from build123d import *

# Parameters (mm, degrees)
SKETCH1_W           = 225.40000005
SKETCH1_H           = 111.10000005
SKETCH1_R           = 2.499999953
BOSS_EXTRUDE1_DEPTH = 19.38655
CUT_EXTRUDE1_DEPTH  = 2.54


with BuildPart() as part:
    # Sketch1 → Boss-Extrude1 (new, symmetric)
    with BuildSketch(Plane(origin=(0, 0, 0), x_dir=(1, 0, 0), z_dir=(0, 1, 0))):
        with Locations((112.700000025, 55.550000025)):
            Rectangle(SKETCH1_W, SKETCH1_H)
        with Locations(Location((4.800000052, 4.800000052, 0), (0, 0, 270))):
            Circle(SKETCH1_R, mode=Mode.SUBTRACT)
        with Locations(Location((4.800000052, 106.400000052, 0), (0, 0, 270))):
            Circle(SKETCH1_R, mode=Mode.SUBTRACT)
        with Locations(Location((220.700000052, 106.400000052, 0), (0, 0, 270))):
            Circle(SKETCH1_R, mode=Mode.SUBTRACT)
        with Locations(Location((220.700000052, 4.800000052, 0), (0, 0, 270))):
            Circle(SKETCH1_R, mode=Mode.SUBTRACT)
    extrude(amount=BOSS_EXTRUDE1_DEPTH, both=True)

    # Sketch2 → Cut-Extrude1 (cut)
    # profile 1 of 3: a face of its own
    with BuildSketch(Plane(origin=(0, 19.38655, 0), x_dir=(1, 0, 0), z_dir=(0, 1, 0))):
        with BuildLine():
            add(Edge.make_bspline(
                [(93.6654446, 62.638119725), (93.65621175, 62.255926888), (93.637663033, 61.488104777), (93.466421809, 60.341834085), (93.201255703, 59.201705874), (92.836997723, 58.075217304), (92.359286935, 56.979010165), (91.762331794, 55.932624231), (91.032595392, 54.955716054), (90.207106522, 54.027487516), (89.252652089, 53.179116743), (88.173798237, 52.414727304), (86.973600637, 51.734204765), (85.655660468, 51.128628725), (84.202701193, 50.653409294), (82.618753702, 50.300761726), (80.898189452, 50.099121533), (79.705954978, 50.07473573), (79.09029785, 50.062143162)],
                knots=[0, 0, 0, 0, 0.84837333, 1.704374698, 2.568122001, 3.446177459, 4.329841521, 5.219461111, 6.115085959, 7.03322926, 7.973947317, 8.94447037, 9.964314875, 11.034235969, 12.160282575, 13.352588404, 14.632904974, 16, 16, 16, 16], degree=3))
            Line((79.09029785, 50.062143162), (74.528088962, 50.062143162))
            Line((74.528088962, 50.062143162), (74.528088962, 36.39260342))
            Line((74.528088962, 36.39260342), (69.060273065, 36.39260342))
            Line((69.060273065, 36.39260342), (69.060273065, 74.120533108))
            Line((69.060273065, 74.120533108), (79.611449053, 74.120533108))
            add(Edge.make_bspline(
                [(79.611449053, 74.120533108), (80.070260309, 74.115673927), (80.980958213, 74.106028903), (82.329353652, 73.976911734), (83.651671763, 73.795021467), (84.937147693, 73.523102459), (86.171480276, 73.166358976), (87.344146306, 72.730911072), (88.422755699, 72.162952721), (89.43560104, 71.526521333), (90.368402205, 70.791840353), (91.189022047, 69.939252772), (91.912770344, 68.989458848), (92.539599198, 67.944691466), (93.055694596, 66.787250357), (93.402550005, 65.504823346), (93.635402669, 64.110350409), (93.655195832, 63.140369447), (93.6654446, 62.638119725)],
                knots=[0, 0, 0, 0, 1.071095419, 2.126025337, 3.160633674, 4.187194637, 5.191188192, 6.159546808, 7.102471747, 8.032359578, 8.950543616, 9.867691343, 10.788184798, 11.733733012, 12.707489344, 13.737062018, 14.82826569, 16, 16, 16, 16], degree=3))
        make_face()
        with BuildLine():
            add(Edge.make_bspline(
                [(88.197628703, 62.347642005), (88.192174404, 62.63850916), (88.18154377, 63.205420092), (88.067270065, 64.026417972), (87.887321266, 64.795998376), (87.642204989, 65.513494356), (87.324445545, 66.181041679), (86.9271256, 66.789508742), (86.462833318, 67.351595169), (85.92370252, 67.854044286), (85.320326107, 68.296325862), (84.670815804, 68.696121206), (83.954231053, 69.019190265), (83.180431142, 69.281086893), (82.353689397, 69.498799431), (81.465989989, 69.635809834), (80.527957319, 69.737538529), (79.882297045, 69.743319744), (79.551644817, 69.74628039)],
                knots=[0, 0, 0, 0, 1.07893025, 2.102875295, 3.069403633, 4.00867391, 4.911619206, 5.805799344, 6.69897942, 7.61127936, 8.532960211, 9.47193309, 10.436783978, 11.442898866, 12.50165651, 13.605056338, 14.773513735, 16, 16, 16, 16], degree=3))
            Line((79.551644817, 69.74628039), (74.528088962, 69.74628039))
            Line((74.528088962, 69.74628039), (74.528088962, 54.43639588))
            Line((74.528088962, 54.43639588), (79.115928237, 54.43639588))
            add(Edge.make_bspline(
                [(79.115928237, 54.43639588), (79.469215163, 54.444058583), (80.154049634, 54.458912469), (81.153694325, 54.542163566), (82.091850755, 54.691905292), (82.964265919, 54.917155421), (83.774695488, 55.18910777), (84.524586407, 55.521306188), (85.210072438, 55.925895812), (85.836535364, 56.387055958), (86.399655255, 56.909209561), (86.877940326, 57.506401351), (87.291847487, 58.157818385), (87.628287432, 58.875259995), (87.880108968, 59.657394144), (88.069138486, 60.497611643), (88.18153711, 61.401962584), (88.192147378, 62.025512532), (88.197628703, 62.347642005)],
                knots=[0, 0, 0, 0, 1.232805628, 2.389751021, 3.4973379, 4.54330244, 5.530003372, 6.477393866, 7.399377973, 8.301660217, 9.187431021, 10.070466494, 10.963674817, 11.874940633, 12.827061481, 13.825105319, 14.876436953, 16, 16, 16, 16], degree=3))
        make_face(mode=Mode.SUBTRACT)
    # profile 2 of 3: a face of its own
    with BuildSketch(Plane(origin=(0, 19.38655, 0), x_dir=(1, 0, 0), z_dir=(0, 1, 0))):
        with BuildLine():
            add(Edge.make_bspline(
                [(127.56590316, 55.675197919), (127.547617612, 54.78857119), (127.511689457, 53.046492477), (127.23969054, 50.905769989), (126.922569652, 49.262016243), (126.614411717, 48.087206761), (126.246431872, 46.950715858), (125.811824352, 45.860819894), (125.314265868, 44.812615172), (124.753130965, 43.8086857), (124.107420568, 42.863739226), (123.409082848, 41.959258432), (122.626828334, 41.117422828), (121.7596775, 40.338177311), (120.809466051, 39.618619159), (119.771337822, 38.967548349), (118.647283346, 38.391422091), (117.447711896, 37.861858683), (116.153140186, 37.424384305), (114.773384937, 37.046415803), (113.301688648, 36.744518404), (111.730514486, 36.548407326), (110.065508535, 36.414654635), (108.921503761, 36.400080642), (108.334569436, 36.39260342)],
                knots=[0, 0, 0, 0, 1.874627119, 3.68334034, 4.55511198, 5.414139205, 6.25033141, 7.080252411, 7.893905149, 8.703019486, 9.509911256, 10.312362027, 11.117881282, 11.936734267, 12.775179546, 13.635831221, 14.524848569, 15.444673208, 16.406604644, 17.411911457, 18.469143348, 19.580838344, 20.758843452, 22, 22, 22, 22], degree=3))
            Line((108.334569436, 36.39260342), (100.226823676, 36.39260342))
            Line((100.226823676, 36.39260342), (100.226823676, 74.120533108))
            Line((100.226823676, 74.120533108), (109.983457667, 74.120533108))
            add(Edge.make_bspline(
                [(109.983457667, 74.120533108), (110.698796565, 74.108775888), (112.087312401, 74.085954417), (114.099407103, 73.871359676), (115.971010991, 73.513186255), (117.705932553, 73.024742171), (119.296694788, 72.37897733), (120.753078111, 71.603929555), (122.063935524, 70.672214529), (123.234870408, 69.595919293), (124.268375898, 68.375042443), (125.15212849, 66.998343044), (125.905974417, 65.477332321), (126.520334079, 63.804439371), (126.984079723, 61.979297568), (127.323005556, 60.011417912), (127.529971236, 57.892365797), (127.553664927, 56.430354144), (127.56590316, 55.675197919)],
                knots=[0, 0, 0, 0, 1.17177347, 2.274482801, 3.310388109, 4.291013938, 5.222472681, 6.118087065, 6.988127256, 7.850034114, 8.717518086, 9.601485366, 10.523818561, 11.493740021, 12.515690363, 13.604990885, 14.762933224, 16, 16, 16, 16], degree=3))
        make_face()
        with BuildLine():
            add(Edge.make_bspline(
                [(122.098087263, 55.239481339), (122.091167759, 55.883338842), (122.07786261, 57.121378364), (121.941863816, 58.899207539), (121.714490077, 60.523833747), (121.395141619, 62.00003254), (120.973701982, 63.330931753), (120.478179626, 64.534888844), (119.856705316, 65.588603714), (119.150728012, 66.521049001), (118.340699821, 67.317635038), (117.439068976, 68.005524695), (116.438452675, 68.568612468), (115.337592989, 69.003716428), (114.147410598, 69.331977904), (112.863376849, 69.585308184), (111.475458259, 69.713259964), (110.519060263, 69.735050507), (110.026174979, 69.74628039)],
                knots=[0, 0, 0, 0, 1.413547595, 2.71803587, 3.911871408, 5.013341294, 6.029850817, 6.974090411, 7.865305992, 8.708270035, 9.535123508, 10.351794371, 11.191784495, 12.047569406, 12.944296091, 13.8996306, 14.91756238, 16, 16, 16, 16], degree=3))
            Line((110.026174979, 69.74628039), (105.694639573, 69.74628039))
            Line((105.694639573, 69.74628039), (105.694639573, 40.766856138))
            Line((105.694639573, 40.766856138), (109.462306464, 40.766856138))
            add(Edge.make_bspline(
                [(109.462306464, 40.766856138), (109.972390662, 40.779628967), (110.963897054, 40.804456912), (112.404673192, 40.959074575), (113.741396992, 41.254449715), (114.982492322, 41.645412228), (116.128283102, 42.146846942), (117.168651881, 42.778873861), (118.119824521, 43.514260641), (118.95603885, 44.379608434), (119.710984868, 45.341779056), (120.348177326, 46.429272224), (120.897700383, 47.621563924), (121.340339899, 48.927882581), (121.678563879, 50.347150333), (121.924720399, 51.877582623), (122.068484344, 53.522343822), (122.088017719, 54.655390557), (122.098087263, 55.239481339)],
                knots=[0, 0, 0, 0, 1.112402768, 2.162298815, 3.153767855, 4.092494856, 4.996014567, 5.873553179, 6.740614794, 7.610074679, 8.4907496, 9.401305331, 10.351566166, 11.349161427, 12.403455731, 13.529502205, 14.72644707, 16, 16, 16, 16], degree=3))
        make_face(mode=Mode.SUBTRACT)
    # profile 3 of 3: a face of its own
    with BuildSketch(Plane(origin=(0, 19.38655, 0), x_dir=(1, 0, 0), z_dir=(0, 1, 0))):
        Polygon((158.732453771, 36.39260342), (153.264637875, 36.39260342), (153.264637875, 53.88961429), (137.954753364, 53.88961429), (137.954753364, 36.39260342), (132.486937467, 36.39260342), (132.486937467, 74.120533108), (137.954753364, 74.120533108), (137.954753364, 58.263867007), (153.264637875, 58.263867007), (153.264637875, 74.120533108), (158.732453771, 74.120533108), align=None)
    extrude(amount=-CUT_EXTRUDE1_DEPTH, mode=Mode.SUBTRACT)


solid = part.part
CAD build for the part. Positions are in the model's coordinates, mm. Coordinates: 2 decimals unless noted, no trailing zeros. Order: outer loops, then holes, each group sorted by start corner. A loop starts at its lowest first (then second) coordinate and runs counter-clockwise, first axis right, second up.
Item 1: Band-saw the part on B-B on z = -4.8. List the corners of the cut face in (x, y), plus the area to 3 significant figures.
Check sheet entries:
outline: (0, -19.39) - (2.3, -19.39) - (2.3, 19.39) - (0, 19.39) - close; (7.3, -19.39) - (218.2, -19.39) - (218.2, 19.39) - (7.3, 19.39) - close; (223.2, -19.39) - (225.4, -19.39) - (225.4, 19.39) - (223.2, 19.39) - close
area: 8,350 mm2
Item 2: Drill centre lines: L1, parallel to X at y = -7, z = -106; L2, parallel to Z at x = 79, y = 18; L3, parallel to Z at x = 4, y = 1. Where is each one in solid material? Low to high.
Check sheet entries:
L1: x = 0 to 2.33, 7.27 to 218.23, 223.17 to 225.4
L2: z = -111.1 to -74.12, -69.75 to -54.44, -50.06 to 0
L3: z = -111.1 to -108.77, -104.03 to -7.17, -2.43 to 0
Item 3: Two-plate mould, pull along X, no slides. Class faces 1 (the face through (0, 0, -55)), 2 (the face through (73, 16.847, -60)), 3 (the face through (114, 19.387, -55)): +X half, -X half, draft (parallel to the pull), parting line (faces both ways), or undercut.
Check sheet entries:
face 1: -X half
face 2: undercut
face 3: draft
Item 4: Band-saw the part on A-A on x = 4.8. List the corners of the cut face in (y, z).
Check sheet entries:
outline: (-19.39, -111.1) - (19.39, -111.1) - (19.39, -108.9) - (-19.39, -108.9) - close; (-19.39, -103.9) - (19.39, -103.9) - (19.39, -7.3) - (-19.39, -7.3) - close; (-19.39, -2.3) - (19.39, -2.3) - (19.39, 0) - (-19.39, 0) - close
